```python
from build123d import *

# Parameters (mm, degrees)
SKETCH_1_W        = 246
SKETCH_1_H        = 98
EXTRUDE_1_DEPTH   = 1
SKETCH_2_W        = 246
SKETCH_2_H        = 1
EXTRUDE_2_DEPTH   = 11
HOLE_WIZARD_M41_D = 4.2


with BuildPart() as part:
    # Эскиз1 → Бобышка-Вытянуть1 (new body)
    with BuildSketch(Plane(origin=(0, 0, 0), x_dir=(1, 0, 0), z_dir=(0, 1, 0))):
        Rectangle(SKETCH_1_W, SKETCH_1_H)
    extrude(amount=EXTRUDE_1_DEPTH)

    # Эскиз2 → Бобышка-Вытянуть2 (add)
    with BuildSketch(Plane.XZ):
        with Locations((0, 48.5)):
            Rectangle(SKETCH_2_W, SKETCH_2_H)
    extrude(amount=EXTRUDE_2_DEPTH)

    # Сверло под метчик  спиральное M41 (through all)
    with Locations(Plane.XY.offset(49)):
        with Locations((118.5, -5), (-118.5, -5)):
            Hole(HOLE_WIZARD_M41_D / 2)


solid = part.part
```
CAD build for the part. Positions are in the model's coordinates, mm. A direction names the side the tool comes from. Give positions to 0.01 mm unless a question says otherwise; leave off trailing zeros. Order: outer loops, then holes, each group sorted by start corner. A loop starts at its lowest first (then second) coordinate and runs counter-clockwise, first axis right, second up.
(1) Saw through at C-C, the plane z = 28. Give the cut face in (x, y).
(2) Tool access for faces 4 (the flat face through (-2, -5, 48)), 5 (the cylindrical face through (-120.44, -5.8, 48.49)): list every direction of +Z, -Z, +X, -X, +Y, -Y with a clear straight run to the whole face (end or side of a thin tool).
(3) Saw through at A-A, the plane y = -5. Give the cut face in (x, z), then the cut area to 3 significant figures.
(4) Drill centre lines: L1, parallel to Y at x = 118.5, z = 48.7; L2, parallel to Y at x = -109, z = 18.5; L3, parallel to Z at x = -110, y = -0.25. Where is each one in solid material? Low to high.
(5) Saw through at B-B, the plane x = -90. Give the cut face in (y, z).
(6) Flat gauge pins, fed straight in: pin 1 (8 mm diameter, centred on x = 13, z = 25, fed in from -Y); pin 2 (6 mm diameter, centred on y = -3.5, z = 17, fed in from +X); pin 3 (5 mm diameter, centred on x = -118.5, y = -5, fed in from -Z); pin 4 (4 mm diameter, centred on x = -6.5, y = -1, fed in from -Z). Where does each tip first touch, or does it go through?
(7) Mould opens along X. For faces 1 (the cylindrical face through (116.56, -5.8, 48.49)), 2 (the flat face through (-2, 0, -1)), 3 (the flat face through (-123, 0.8, -0.2)) say: released by +X, released by -X, zero draft, split by the parting line, or undercut.
Results found:
1. outline: (-123, 0) - (123, 0) - (123, 1) - (-123, 1) - close
2. face 4: -Z, +X, -X, -Y
2. face 5: +Z, -Z
3. outline: (-123, 48) - (-120.6, 48) - (-120.6, 49) - (-123, 49) - close; (-116.4, 48) - (116.4, 48) - (116.4, 49) - (-116.4, 49) - close; (120.6, 48) - (123, 48) - (123, 49) - (120.6, 49) - close
3. area: 238 mm2
4. L1: y = -11 to -7.1, -2.9 to 1
4. L2: y = 0 to 1
4. L3: z = 48 to 49
5. outline: (-11, 48) - (0, 48) - (0, -49) - (1, -49) - (1, 49) - (-11, 49) - close
6. pin 1: stops at y = 0
6. pin 2: passes through
6. pin 3: stops at z = 48
6. pin 4: stops at z = -49
7. face 1: undercut
7. face 2: zero draft
7. face 3: released by -X
